Build history of the part. All positions in model axes, mm. Face numbers are marked on the shaded views. A direction names the side the tool comes from. Round coordinates to 2 decimals unless told otherwise and drop trailing zeros. Write each loop counter-clockwise with the first axis right and the second up, starting at its lowest first coordinate (ties: lowest second). Pieces come first, ordered by that corner, then holes. Notation, with made-up numbers: M 84,-34 L 108,-34 A31 cw 108,2 Z; hole C -10.75,-29 d11. An arc over 180 degrees is marked long. Use a Markdown table: item, result.
from build123d import *

# Parameters (mm, degrees)
F0_R     = 40
F1_DEPTH = 98.2
F3_DEPTH = 100
F5_R     = 8
F6_DEPTH = 200
F8_R     = 8
F9_DEPTH = 100


with BuildPart() as f1:
    # F0 (on Top) → F1 (new body)
    with BuildSketch(Plane.XY):
        Circle(F0_R)
    extrude(amount=F1_DEPTH)

    # F2 (on face) → F3 (cut)
    with BuildSketch(Plane.XY.offset(98.2)):
        Polygon((26.884189, -0.158689), (13.579523, 23.203046), (-13.304666, 23.361735), (-26.884189, 0.158689), (-13.579523, -23.203046), (13.304666, -23.361735), align=None)
    extrude(amount=-F3_DEPTH, mode=Mode.SUBTRACT)

    # F5 (on offset) → F6 (cut)
    with BuildSketch(Plane.XZ.offset(45)):
        with Locations((0, 99.055015)):
            Circle(F5_R)
    extrude(amount=-F6_DEPTH, mode=Mode.SUBTRACT)

    # F8 (on offset) → F9 (cut)
    with BuildSketch(Plane.YZ.offset(50)):
        with Locations((0, 98.486878)):
            Circle(F8_R)
    extrude(amount=-F9_DEPTH, mode=Mode.SUBTRACT)


solid = f1.part
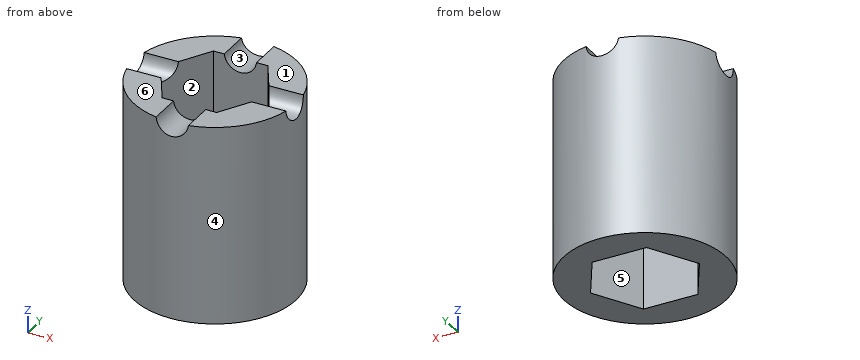
Q1. Two-plate mould, pull along X, no slides. Class the marked faces 1, 2, 3 and 4: +X half, -X half, draft (parallel to the pull), parting line (faces both ways), or undercut.
Response values:
| item | result |
|---|---|
| face 1 | draft |
| face 2 | undercut |
| face 3 | undercut |
| face 4 | parting line |
Q2. Drill centre lines: L1, parallel to Y at x = -12, z = 58; L2, parallel to X at y = -7, z = 11; L3, parallel to X at y = 9.5, z = 56.5. Where is each one in solid material? Low to high.
Response values:
| item | result |
|---|---|
| L1 | y = -38.16 to -23.21, 23.35 to 38.16 |
| L2 | x = -39.38 to -22.81, 22.88 to 39.38 |
| L3 | x = -38.86 to -21.42, 21.38 to 38.86 |
Q3. Cut at A-A on z = 15. Give the cut face in (x, y), and give its area (3 significant figures).
Response values:
| item | result |
|---|---|
| outline | C 0,0 d80; hole M -26.88,0.16 L -13.58,-23.2 L 13.3,-23.36 L 26.88,-0.16 L 13.58,23.2 L -13.3,23.36 Z |
| area | 3,150 mm2 |
Q4. Cut at D-D on x = -24. Give the cut face in (y, z).
Response values:
| item | result |
|---|---|
| outline | M -32,0 L -4.91,0 L -4.91,92.17 A8 cw -7.99,98.2 L -32,98.2 Z; M 5.09,0 L 32,0 L 32,98.2 L 7.99,98.2 A8 cw 5.09,92.31 Z |
Q5. Drop flat-ended pins along their axis: P1, Ø8, axis at x = -14, z = 44.5, coming from the +Y side; P2, Ø1, axis at x = -25, z = 38.5, coming from the -Y side; P3, Ø10, axis at y = -23, z = 30.5, coming from the +X side. Give the stop position or say it passes through.
Response values:
| item | result |
|---|---|
| P1 | stops at y = 38.73 |
| P2 | stops at y = -31.62 |
| P3 | stops at x = 35.72 |
Q6. Which spindle directions (+Z, -Z, +X, -X, +Y, -Y) get a long thin tool onto all of the face, cutting with end or side? Do the marked faces 5 and 6. Say none if no direction does.
Response values:
| item | result |
|---|---|
| face 5 | +Z, -Z |
| face 6 | +Z, +X, -X, +Y, -Y |
Q7. Cut at C-C on x = 17.5. Give the cut face in (y, z).
Response values:
| item | result |
|---|---|
| outline | M -35.97,0 L -16.19,0 L -16.19,98.2 L -35.97,98.2 Z; M 16.32,0 L 35.97,0 L 35.97,98.2 L 16.32,98.2 Z |
Q8. Cut at B-B on y = -6.5. Give the cut face in (x, z), and give its area (3 significant figures).
Response values:
| item | result |
|---|---|
| outline | M -39.47,0 L -23.09,0 L -23.09,93.82 L -39.47,93.82 Z; M 23.17,0 L 39.47,0 L 39.47,93.82 L 23.17,93.82 Z |
| area | 3,070 mm2 |
